Design review of the part built by this model. Coordinates are the model's own, in mm. Face numbers are marked on the shaded views. A direction names the side the tool comes from. Coordinates: 2 decimals unless noted, no trailing zeros. Loops run counter-clockwise (first coordinate to the right, second up) from the corner with the lowest first, then second, coordinate; pieces in that order, holes last. Notation, with made-up numbers: (-12, 75) -> (10, 75) arc R17 ccw to (10, 89) -> close; hole circle Ø8 at (48, 1). An arc over 180 degrees is marked (long way). One line per item, written item: value. Start each with the question number.
1. Add section A-A on x = 13.25. Write out the cut boundary in (y, z).
2. Machinability: for the marked faces 1, 2, 3, 4 and 5, which of the approach directions +Z, -Z, +X, -X, +Y, -Y give a long, thin tool a straight path to every point of the face, cutting with its end or side? Answer none if there is none.
3. Add section B-B on z = 0. Write out the cut boundary in (x, y).
4. Add section D-D on y = -11. Write out the cut boundary in (x, z), plus the area to 3 significant figures.
5. Add section C-C on y = 1.25. Write out the cut boundary in (x, z), plus the area to 3 significant figures.
6. Draft analysis for pull direction Y (two halves, no side actions). For the marked faces 6, 7 and 8, state which applies: pulls with the +Y half, pulls with the -Y half, needs draft (parallel to the pull), parting line crosses it, or undercut.
7. Insertion check: pin 1 (8 mm diameter, centred on y = 0, z = 0, fed in from -X); pin 2 (12 mm diameter, centred on x = 6, y = 5, fed in from -Z); pin 3 (9 mm diameter, centred on x = 5, z = 5, fed in from +Y); pin 4 (1 mm diameter, centred on x = 7.5, y = 7, fed in from -Z). Each pin has a flat end and moves straight along its axis. Give the tip position at first contact, or say it passes through.
8. For probe 1 along Z at (x, y) = (5, -7.9); probe 2 along Z at (x, y) = (15.75, -2); probe 3 along Y at (x, z) = (3, 0.25), list the stretches that pass through material, from the lowest coordinate up.
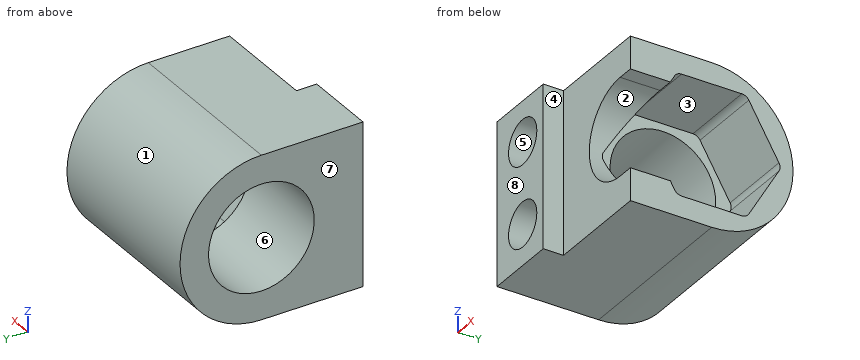
```python
from build123d import *

# Parameters (mm, degrees)
SKIZZE1_R                       = 6.5
AUFSATZ_LINEAR_AUSTRAGEN1_DEPTH = 22
SCHNITT_LINEAR_AUSTRAGEN1_DEPTH = 9.5
SKIZZE3_R                       = 2.75
SCHNITT_LINEAR_AUSTRAGEN2_DEPTH = 6
SCHNITT_LINEAR_AUSTRAGEN3_REACH = 24.5
SKIZZE5_W                       = 13
SKIZZE5_H                       = 20
SCHNITT_LINEAR_AUSTRAGEN4_DEPTH = 2.5


with BuildPart() as part:
    # Skizze1 → Aufsatz-Linear austragen1 (new body)
    with BuildSketch(Plane(origin=(0, 0, 0), x_dir=(0, 0, -1), z_dir=(1, 0, 0))):
        with BuildLine():
            Line((-10, 0), (-10, -12.5))
            Line((-10, -12.5), (10, -12.5))
            Line((10, -12.5), (10, 0))
            ThreePointArc((10, 0), (0, 10), (-10, 0))
        make_face()
        Circle(SKIZZE1_R, mode=Mode.SUBTRACT)
    extrude(amount=AUFSATZ_LINEAR_AUSTRAGEN1_DEPTH)

    # Skizze2 → Schnitt-Linear austragen1 (cut)
    with BuildSketch(Plane(origin=(22, 0, 0), x_dir=(0, 0, -1), z_dir=(1, 0, 0))):
        with BuildLine():
            Line((7.410637894, -3.701183514), (7.410637894, 3.701183514))
            ThreePointArc((7.410637894, 3.701183514), (7.276663298, 4.201183514), (6.910637894, 4.567208918))
            Line((6.910637894, 4.567208918), (0.5, 8.268392432))
            ThreePointArc((0.5, 8.268392432), (0, 8.402367028), (-0.5, 8.268392432))
            Line((-0.5, 8.268392432), (-6.910637894, 4.567208918))
            ThreePointArc((-6.910637894, 4.567208918), (-7.276663298, 4.201183514), (-7.410637894, 3.701183514))
            Line((-7.410637894, 3.701183514), (-7.410637894, -3.701183514))
            ThreePointArc((-7.410637894, -3.701183514), (-7.276663298, -4.201183514), (-6.910637894, -4.567208918))
            Line((-6.910637894, -4.567208918), (-0.5, -8.268392432))
            ThreePointArc((-0.5, -8.268392432), (0, -8.402367028), (0.5, -8.268392432))
            Line((0.5, -8.268392432), (6.910637894, -4.567208918))
            ThreePointArc((6.910637894, -4.567208918), (7.276663298, -4.201183514), (7.410637894, -3.701183514))
        make_face()
    extrude(amount=-SCHNITT_LINEAR_AUSTRAGEN1_DEPTH, mode=Mode.SUBTRACT)

    # Skizze3 → Schnitt-Linear austragen2 (cut)
    with BuildSketch(Plane.XZ.offset(12.5)):
        with Locations((5, 5)):
            Circle(SKIZZE3_R)
        with Locations((5, -5)):
            Circle(SKIZZE3_R)
    extrude(amount=-SCHNITT_LINEAR_AUSTRAGEN2_DEPTH, mode=Mode.SUBTRACT)

    # Skizze4 → Schnitt-Linear austragen3 (cut, up to next)
    with BuildSketch(Plane.XZ.offset(12.5), mode=Mode.PRIVATE) as schnitt_linear_austragen3_sk1:
        with BuildLine():
            Line((20, 6), (22, 6))
            Line((22, 6), (22, -6))
            Line((22, -6), (20, -6))
            ThreePointArc((20, -6), (14, 0), (20, 6))
        make_face()
    schnitt_linear_austragen3_tool1 = extrude(schnitt_linear_austragen3_sk1.sketch, amount=-SCHNITT_LINEAR_AUSTRAGEN3_REACH, mode=Mode.PRIVATE) & part.part
    add(schnitt_linear_austragen3_tool1.solids().sort_by_distance((18.510217, -12.5, 0))[0], mode=Mode.SUBTRACT)

    # Skizze5 → Schnitt-Linear austragen4 (cut)
    with BuildSketch(Plane.XZ.offset(12.5)):
        with Locations((15.5, 0)):
            Rectangle(SKIZZE5_W, SKIZZE5_H)
    extrude(amount=-SCHNITT_LINEAR_AUSTRAGEN4_DEPTH, mode=Mode.SUBTRACT)


solid = part.part
```
Worked answers:
1. outline: (-10, -10) -> (0, -10) arc R10 ccw to (0, 10) -> (-10, 10) -> close; hole (-8.27, -0.5) -> (-4.57, -6.91) arc R1 ccw to (-3.7, -7.41) -> (3.7, -7.41) arc R1 ccw to (4.57, -6.91) -> (8.27, -0.5) arc R1 ccw to (8.27, 0.5) -> (4.57, 6.91) arc R1 ccw to (3.7, 7.41) -> (-3.7, 7.41) arc R1 ccw to (-4.57, 6.91) -> (-8.27, 0.5) arc R1 ccw to start
2. face 1: +X, -X, +Y
2. face 2: +X, -Y
2. face 3: +X
2. face 4: +Z, -Z, +X, -Y
2. face 5: -Y
3. outline: (0, -12.5) -> (9, -12.5) -> (9, -10) -> (14, -10) -> (14, -8.4) -> (12.5, -8.4) -> (12.5, -6.5) -> (0, -6.5) -> close; (0, 6.5) -> (12.5, 6.5) -> (12.5, 8.4) -> (22, 8.4) -> (22, 10) -> (0, 10) -> close
4. outline: (0, -10) -> (9, -10) -> (9, 10) -> (0, 10) -> close; hole circle Ø5.5 at (5, -5); hole circle Ø5.5 at (5, 5)
4. area: 132 mm²
5. outline: (0, -9.92) -> (22, -9.92) -> (22, -7.41) -> (12.5, -7.41) -> (12.5, -6.38) -> (0, -6.38) -> close; (0, 6.38) -> (12.5, 6.38) -> (12.5, 7.41) -> (22, 7.41) -> (22, 9.92) -> (0, 9.92) -> close
5. area: 136 mm²
6. face 6: undercut
6. face 7: needs draft
6. face 8: pulls with the -Y half
7. pin 1: passes through
7. pin 2: stops at z = -10
7. pin 3: stops at y = 9.99
7. pin 4: stops at z = -7.6
8. probe 1: z = -10 to -7.75, -2.25 to 2.25, 7.75 to 10
8. probe 2: z = -10 to -7.41, 7.41 to 10
8. probe 3: y = -12.5 to -6.5, 6.5 to 10
